Here's how the part is built. I have some questions about the finished solid (model axes, mm). Face numbers are marked on the shaded views. A direction names the side the tool comes from. Coordinates: 2 decimals unless noted, no trailing zeros. Order: outer loops, then holes, each group sorted by start corner. A loop starts at its lowest first (then second) coordinate and runs counter-clockwise, first axis right, second up.
```python
from build123d import *

# Parameters (mm, degrees)
SKETCH1_R           = 3.175
BOSS_EXTRUDE1_DEPTH = 12.7
BOSS_EXTRUDE2_DEPTH = 6.35
SKETCH3_R           = 2.0828
BOSS_EXTRUDE3_DEPTH = 9.525


with BuildPart() as part:
    # Sketch1 → Boss-Extrude1 (new body)
    with BuildSketch(Plane.XY):
        Circle(SKETCH1_R)
    extrude(amount=BOSS_EXTRUDE1_DEPTH)

    # Sketch2 → Boss-Extrude2 (add)
    with BuildSketch(Plane.XY.offset(12.7)):
        Polygon((3.666174209, -6.35), (7.332348419, 0), (3.666174209, 6.35), (-3.666174209, 6.35), (-7.332348419, 0), (-3.666174209, -6.35), align=None)
    extrude(amount=BOSS_EXTRUDE2_DEPTH)

    # Sketch3 → Boss-Extrude3 (add)
    with BuildSketch(Plane.XY.offset(19.05)):
        Circle(SKETCH3_R)
    extrude(amount=BOSS_EXTRUDE3_DEPTH)


solid = part.part
```
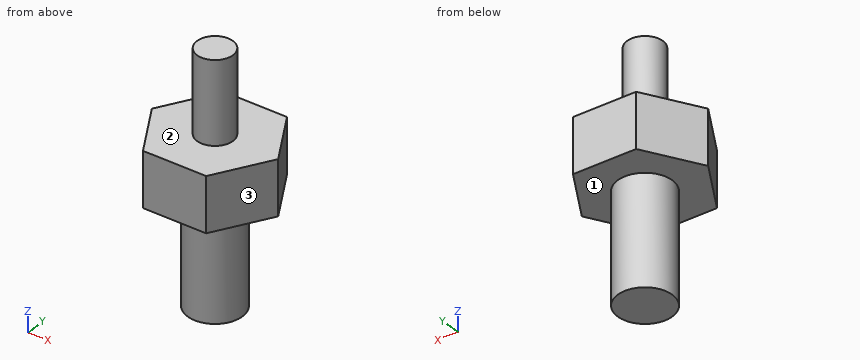
Q1. I need wall thicknesses on L1, parallel to Z at x = 2.75, y = -5.5; L2, parallel to Y at x = 5.5, z = 17.25; L3, parallel to Z at x = -0.25, y = -2.25. Which ranges of each line are inside material? Lowest first, please.
Q2. Will these pins go through, and if not, where does the flat tip stop? pin 1 (5 mm diameter, centred on x = -1.5, z = 25.5, fed in from +Y); pin 2 (6.5 mm diameter, centred on x = 1.5, y = -2, fed in from +Z) (3 decimals); pin 3 (2 mm diameter, centred on x = -2.5, z = 21.5, fed in from +Y) (3 decimals).
Q3. If we section it at B-B on y = -0.5: Write out the boundary of the cut face in (x, z) (3 decimals), then the cut area to 3 significant figures.
Q4. If we section it at A-A on x = 0: Write out the boundary of the cut face in (y, z) (3 decimals).
Q5. For the marked faces 1, 2 and 3, which set-ups out of +Z, -Z, +X, -X, +Y, -Y let a thin tool reach every point of the face, with its end or its side?
Q6. If we section it at D-D on x = 2.5: Write out the boundary of the cut face in (y, z), then the cut area to 3 significant figures.
Q7. If we section it at C-C on z = 26.25: Write out the boundary of the cut face in (x, y), then the cut area to 3 significant figures.
Reply:
1. L1: z = 12.7 to 19.05
1. L2: y = -3.17 to 3.17
1. L3: z = 0 to 19.05
2. pin 1: stops at y = 2.08
2. pin 2: stops at z = 28.575
2. pin 3: stops at y = 1.445
3. outline: (-7.044, 12.7) - (-3.135, 12.7) - (-3.135, 0) - (3.135, 0) - (3.135, 12.7) - (7.044, 12.7) - (7.044, 19.05) - (2.022, 19.05) - (2.022, 28.575) - (-2.022, 28.575) - (-2.022, 19.05) - (-7.044, 19.05) - close
3. area: 208 mm2
4. outline: (-6.35, 12.7) - (-3.175, 12.7) - (-3.175, 0) - (3.175, 0) - (3.175, 12.7) - (6.35, 12.7) - (6.35, 19.05) - (2.083, 19.05) - (2.083, 28.575) - (-2.083, 28.575) - (-2.083, 19.05) - (-6.35, 19.05) - close
5. face 1: -Z
5. face 2: +Z
5. face 3: +Z, -Z, +X, -Y
6. outline: (-6.35, 12.7) - (-1.96, 12.7) - (-1.96, 0) - (1.96, 0) - (1.96, 12.7) - (6.35, 12.7) - (6.35, 19.05) - (-6.35, 19.05) - close
6. area: 130 mm2
7. outline: circle Ø4.17 at (0, 0)
7. area: 13.6 mm2
